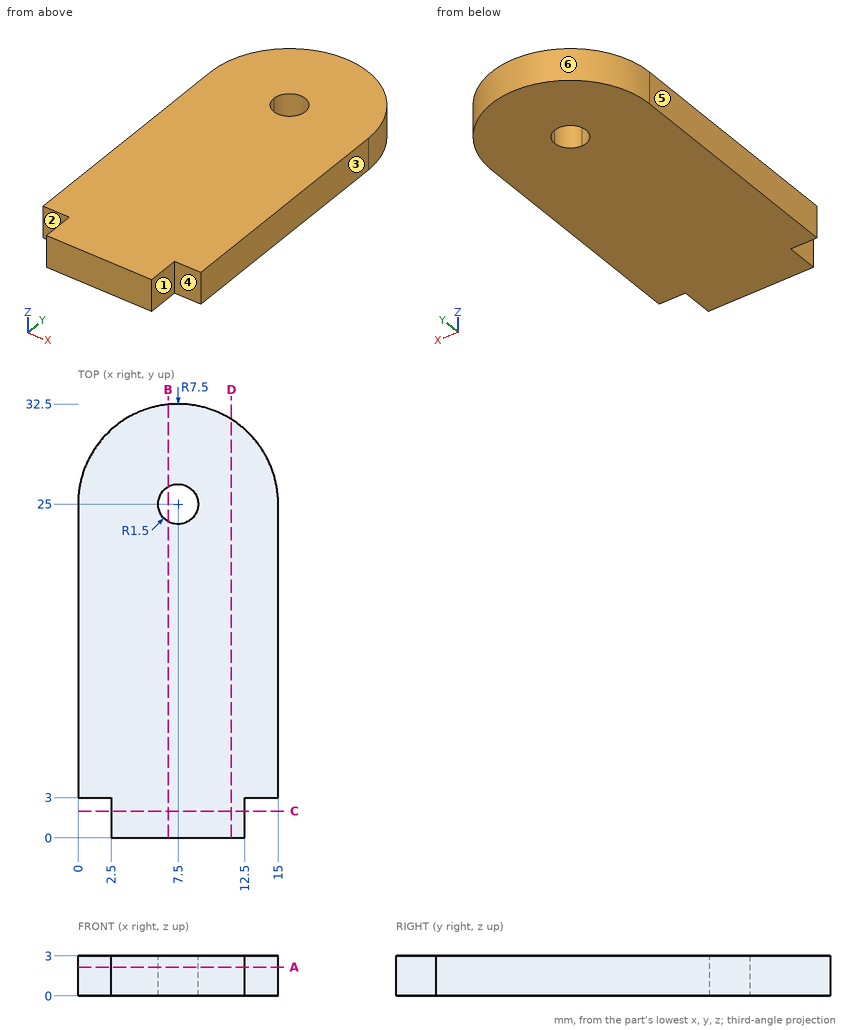
For this review, use the dimensioned drawing (mm, ordinates from the lowest corner) and the shaded views. A direction names the side the tool comes from. Coordinates: 2 decimals unless noted, no trailing zeros. Order: outer loops, then holes, each group sorted by start corner. A loop starts at its lowest first (then second) coordinate and runs counter-clockwise, first axis right, second up. Notation, with made-up numbers: (35.5, 30) -> (86.5, 30) arc R29 cw to (86.5, 63) -> close; hole circle Ø2 at (59.25, -40). An arc over 180 degrees is marked (long way). One line per item, written item: value. Start each with the question number.
Q1. Take a section at C-C, the plane y = 2. State the section outline as (x, z) points, then the cut area to 3 significant figures.
Q2. Insertion check: pin 1 Ø1.2 at (x, z) = (1.5, 1) entering from -Y; pin 2 Ø1.5 at (y, z) = (1.5, 1) entering from -X. Each pin has a flat end and moves straight along its axis. Give the tip position at first contact, or say it passes through.
Q3. Tool access review of the marked faces 1, 2 and 3: name each direction out of +Z, -Z, +X, -X, +Y, -Y from which nothing blocks a thin tool from reaching the whole face with its end or side.
Q4. Take a section at D-D, the plane x = 11.5. State the section outline as (y, z) points, then the cut area to 3 significant figures.
Q5. Take a section at A-A, the plane z = 2.15. State the section outline as (x, y) points, then the cut area to 3 significant figures.
Q6. Mouldability with a two-part tool opening along Y and no side actions: class the marked faces 4, 5 and 6 as pulls with the +Y half, pulls with the -Y half, needs draft (parallel to the pull), parting line crosses it, or undercut.
Q7. For probe 1 along Y at (x, z) = (7.5, 1.4); probe 2 along Y at (x, z) = (6.5, 2.35); probe 3 along Y at (x, z) = (3.25, 0.2), list the stretches that pass through material, from the lowest coordinate up.
Q8. Take a section at B-B, the plane x = 6.75. State the section outline as (y, z) points, then the cut area to 3 significant figures.
Values follow:
1. outline: (2.5, 0) -> (12.5, 0) -> (12.5, 3) -> (2.5, 3) -> close
1. area: 30.0 mm2
2. pin 1: stops at y = 3
2. pin 2: stops at x = 2.5
3. face 1: +Z, -Z, +X, -Y
3. face 2: +Z, -Z, -X, -Y
3. face 3: +Z, -Z, +X, +Y, -Y
4. outline: (0, 0) -> (31.34, 0) -> (31.34, 3) -> (0, 3) -> close
4. area: 94.0 mm2
5. outline: (0, 3) -> (2.5, 3) -> (2.5, 0) -> (12.5, 0) -> (12.5, 3) -> (15, 3) -> (15, 25) arc R7.5 ccw to (0, 25) -> close; hole circle Ø3 at (7.5, 25)
5. area: 441 mm2
6. face 4: pulls with the -Y half
6. face 5: needs draft
6. face 6: pulls with the +Y half
7. probe 1: y = 0 to 23.5, 26.5 to 32.5
7. probe 2: y = 0 to 23.88, 26.12 to 32.43
7. probe 3: y = 0 to 31.18
8. outline: (0, 0) -> (23.7, 0) -> (23.7, 3) -> (0, 3) -> close; (26.3, 0) -> (32.46, 0) -> (32.46, 3) -> (26.3, 3) -> close
8. area: 89.6 mm2
